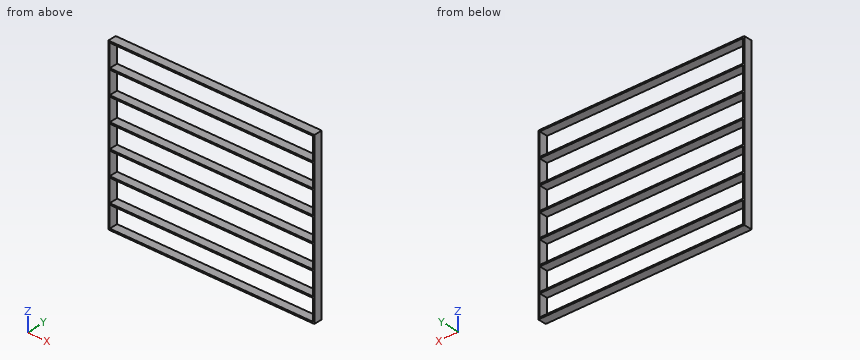
```python
from build123d import *

# Parameters (mm, degrees)
F0_W     = 6.35
F0_H     = 38.1
F1_DEPTH = 755.65
F2_W     = 38.1
F2_H     = 6.35
F3_DEPTH = 457.2


with BuildPart() as f1:
    # F0 (on Top) → F1 (new body)
    with BuildSketch(Plane.XY):
        Rectangle(F0_W, F0_H)
    extrude(amount=F1_DEPTH)

    # F2 (on face) → F3 (join)
    with BuildSketch(Plane.YZ.offset(3.175)):
        with Locations((0, 104.775)):
            Rectangle(F2_W, F2_H)
        with Locations((0, 3.175)):
            Rectangle(F2_W, F2_H)
        with Locations((0, 212.725)):
            Rectangle(F2_W, F2_H)
        with Locations((0, 320.675)):
            Rectangle(F2_W, F2_H)
        with Locations((0, 428.625)):
            Rectangle(F2_W, F2_H)
        with Locations((0, 536.575)):
            Rectangle(F2_W, F2_H)
        with Locations((0, 644.525)):
            Rectangle(F2_W, F2_H)
        with Locations((0, 752.475)):
            Rectangle(F2_W, F2_H)
    extrude(amount=F3_DEPTH)

    # F4: F1 across face


with BuildPart() as f1_1:
    add(f1.part)
    add(f1.part.mirror(Plane(origin=(460.375, 0, 644.525), x_dir=(0, 1, 0), z_dir=(1, 0, 0))))


solid = f1_1.part
```
The model under review builds one solid part; all positions refer to its coordinate system, in mm. Round coordinates to 2 decimals unless told otherwise and drop trailing zeros. Write each loop counter-clockwise with the first axis right and the second up, starting at its lowest first coordinate (ties: lowest second). Pieces come first, ordered by that corner, then holes.
(1) We need section B-B on z = 609. Give the boundary of the cut face in (x, y) (3 decimals), and give its area (3 significant figures).
(2) We need section A-A on x = 520. Give the number of separate pieces and of enclosed holes in the cut face, and give its area (3 significant figures).
(3) Wall thickness on L1, parallel to X at y = -4.5, z = 91 (3 decimals): over which ranges is the line inside the solid? List them lowest first.
Findings below:
1. outline: (-3.175, -19.05) - (3.175, -19.05) - (3.175, 19.05) - (-3.175, 19.05) - close; (917.575, -19.05) - (923.925, -19.05) - (923.925, 19.05) - (917.575, 19.05) - close
1. area: 484 mm2
2. separate pieces: 8
2. enclosed holes: 0
2. area: 1,940 mm2
3. L1: x = -3.175 to 3.175, 917.575 to 923.925
